from build123d import *

# Parameters (mm, degrees)
F0_W      = 78
F0_H      = 50.8
F1_DEPTH  = 38
F3_DEPTH  = 3
F5_DEPTH  = 50.8
F7_DEPTH  = 4.5
F8_R      = 1.5
F9_DEPTH  = 5
F10_W     = 3
F10_H     = 3.25
F11_DEPTH = 4.5
F12_R     = 6
F13_DEPTH = 51
F15_DEPTH = 3
F16_W     = 48.5
F16_H     = 22
F17_DEPTH = 38
F18_SIZE  = 3
F19_R     = 1
F20_DEPTH = 8
F21_R     = 1
F22_DEPTH = 8
F23_R     = 1
F24_DEPTH = 8
F25_R     = 1
F26_DEPTH = 10


with BuildPart() as f1:
    # F0 (on Front) → F1 (new body)
    with BuildSketch(Plane.XZ):
        with Locations((39, 25.4)):
            Rectangle(F0_W, F0_H)
    extrude(amount=F1_DEPTH)

    # F2 (on face) → F3 (cut)
    with BuildSketch(Plane.XY.offset(50.8)):
        with BuildLine():
            Line((70, -2), (8, -2))
            ThreePointArc((8, -2), (6.5857864376, -2.5857864376), (6, -4))
            Line((6, -4), (6, -34))
            ThreePointArc((6, -34), (6.5857864376, -35.4142135624), (8, -36))
            Line((8, -36), (70, -36))
            ThreePointArc((70, -36), (71.4142135624, -35.4142135624), (72, -34))
            Line((72, -34), (72, -4))
            ThreePointArc((72, -4), (71.4142135624, -2.5857864376), (70, -2))
        make_face()
    extrude(amount=-F3_DEPTH, mode=Mode.SUBTRACT)

    # F4 (on face) → F5 (cut, through all)
    with BuildSketch(Plane.XY.offset(50.8)):
        with BuildLine():
            ThreePointArc((62, -2), (54.9289321881, -4.9289321881), (52, -12))
            Line((52, -12), (52, -26))
            ThreePointArc((52, -26), (54.9289321881, -33.0710678119), (62, -36))
            ThreePointArc((62, -36), (68.9507563357, -33.1893662003), (71.9943065333, -26.3373972723))
            ThreePointArc((71.9943065333, -26.3373972723), (75.2, -19), (71.9943065333, -11.6626027277))
            ThreePointArc((71.9943065333, -11.6626027277), (68.9507563357, -4.8106337997), (62, -2))
        make_face()
    extrude(amount=-F5_DEPTH, mode=Mode.SUBTRACT)

    # F6 (on face) → F7 (cut)
    with BuildSketch(Plane.XY.offset(50.8)):
        with BuildLine():
            Line((47.25, -2), (38.75, -2))
            ThreePointArc((38.75, -2), (38.0428932188, -2.2928932188), (37.75, -3))
            Line((37.75, -3), (37.75, -11.5))
            ThreePointArc((37.75, -11.5), (38.0428932188, -12.2071067812), (38.75, -12.5))
            Line((38.75, -12.5), (47.25, -12.5))
            ThreePointArc((47.25, -12.5), (47.9571067812, -12.2071067812), (48.25, -11.5))
            Line((48.25, -11.5), (48.25, -3))
            ThreePointArc((48.25, -3), (47.9571067812, -2.2928932188), (47.25, -2))
        make_face()
    extrude(amount=-F7_DEPTH, mode=Mode.SUBTRACT)

    # F8 (on face) → F9 (cut)
    with BuildSketch(Plane.XY.offset(50.8)):
        with Locations((47, -11.25)):
            Circle(F8_R)
        with Locations((39, -11.25)):
            Circle(F8_R)
        with Locations((39, -3.25)):
            Circle(F8_R)
        with Locations((47, -3.25)):
            Circle(F8_R)
    extrude(amount=-F9_DEPTH, mode=Mode.SUBTRACT)

    # F10 (on face) → F11 (cut)
    with BuildSketch(Plane.XY.offset(50.8)):
        with Locations((39, -1.625)):
            Rectangle(F10_W, F10_H)
    extrude(amount=-F11_DEPTH, mode=Mode.SUBTRACT)

    # F12 (on face) → F13 (cut)
    with BuildSketch(Plane.XY.offset(50.8)):
        with Locations((20.5, -19)):
            Circle(F12_R)
    extrude(amount=-F13_DEPTH, mode=Mode.SUBTRACT)

    # F14 (on face) → F15 (cut)
    with BuildSketch(Plane(origin=(0, 0, 0), x_dir=(1, 0, 0), z_dir=(0, 0, -1))):
        with BuildLine():
            Line((70, 36), (8, 36))
            ThreePointArc((8, 36), (6.5857864376, 35.4142135624), (6, 34))
            Line((6, 34), (6, 4))
            ThreePointArc((6, 4), (6.5857864376, 2.5857864376), (8, 2))
            Line((8, 2), (70, 2))
            ThreePointArc((70, 2), (71.4142135624, 2.5857864376), (72, 4))
            Line((72, 4), (72, 34))
            ThreePointArc((72, 34), (71.4142135624, 35.4142135624), (70, 36))
        make_face()
    extrude(amount=-F15_DEPTH, mode=Mode.SUBTRACT)

    # F16 (on face) → F17 (cut, through all)
    with BuildSketch(Plane.XZ.offset(38)):
        with Locations((24.25, 28)):
            Rectangle(F16_W, F16_H)
    extrude(amount=-F17_DEPTH, mode=Mode.SUBTRACT)

    # F18
    f18_edges = [f1.edges().sort_by_distance(p)[0] for p in [
        (0, -19, 39),
        (0, -19, 17),
    ]]
    chamfer(f18_edges, length=F18_SIZE)

    # F19 (on face) → F20 (cut)
    with BuildSketch(Plane.XY.offset(50.8)):
        with Locations((3, -19)):
            Circle(F19_R)
        with Locations((75, -10)):
            Circle(F19_R)
        with Locations((75, -28)):
            Circle(F19_R)
    extrude(amount=-F20_DEPTH, mode=Mode.SUBTRACT)

    # F21 (on face) → F22 (cut)
    with BuildSketch(Plane(origin=(0, 0, 0), x_dir=(1, 0, 0), z_dir=(0, 0, -1))):
        with Locations((75, 28)):
            Circle(F21_R)
        with Locations((75, 10)):
            Circle(F21_R)
        with Locations((3, 19)):
            Circle(F21_R)
    extrude(amount=-F22_DEPTH, mode=Mode.SUBTRACT)

    # F23 (on face) → F24 (cut)
    with BuildSketch(Plane(origin=(0, 0, 3), x_dir=(1, 0, 0), z_dir=(0, 0, -1))):
        with Locations((41.5, 15)):
            Circle(F23_R)
    extrude(amount=-F24_DEPTH, mode=Mode.SUBTRACT)

    # F25 (on face) → F26 (cut)
    with BuildSketch(Plane.YZ.offset(78)):
        with Locations((-26.7781745931, 34.7781745931)):
            Circle(F25_R)
        with Locations((-11.2218254069, 34.7781745931)):
            Circle(F25_R)
        with Locations((-26.7781745931, 19.2218254069)):
            Circle(F25_R)
        with Locations((-11.2218254069, 19.2218254069)):
            Circle(F25_R)
    extrude(amount=-F26_DEPTH, mode=Mode.SUBTRACT)


solid = f1.part
Geometry: final body of the model. Coordinates: model frame, mm. A direction names the side the tool comes from. Coordinates: 2 decimals unless noted, no trailing zeros. Loops run counter-clockwise (first coordinate to the right, second up) from the corner with the lowest first, then second, coordinate; pieces in that order, holes last. Notation, with made-up numbers: M 25,-25.5 L 32,-25.5 A20 cw 32,-3.5 Z; hole C 58.25,-40 d1. An arc over 180 degrees is marked long. One line per item, written item: value. Start each with the question number.
1) Draft query along Y for faces 5 (the flat face through (6, -19, 1)), 6 (the flat face through (0, -19, 7)). Return one class per face: released by +Y, released by -Y, zero draft, split by the parting line, or undercut.
2) Cut plane C-C (y = -30). Return loops of the section in (x, z), then the cut area to 3 significant figures.
3) Material intervals for L1, parallel to Y at x = 39, z = 46; L2, parallel to Z at x = 47.5, y = -10; L3, parallel to X at y = -28, z = 4, sorted ascending. Write a range as from..to.
4) Pin query (flat end, axial travel): P1, Ø6, axis at y = -22.5, z = 18.5, coming from the -X side; P2, Ø1, axis at x = 28, z = 45.5, coming from the +Y side; P3, Ø1.5, axis at x = 39, y = -11, coming from the +Z side; P4, Ø3, axis at x = 45, y = -5, coming from the +Z side. Return the tip coordinate at first contact, or that it passes through.
5) Reachability of faces 1 (the flat face through (70, -4, 47.8)), 2 (the flat face through (25.4, -23.5, 17)), 3 (the flat face through (40.5, -1, 49)), 4 (the flat face through (72, -30, 1)) from +Z, -Z, +X, -X, +Y, -Y: full face, straight path, thin tool, end or side. Return the list, or none.
6) Cut plane A-A (x = 47). Return loops of the section in (y, z).
7) Cut plane D-D (x = 20.5). Return loops of the section in (y, z), then the cut area to 3 significant figures.
Evaluation:
1. face 5: undercut
1. face 6: zero draft
2. outline: M 0,0 L 6,0 L 6,3 L 52.83,3 L 52.83,47.8 L 6,47.8 L 6,50.8 L 0,50.8 L 0,42 L 3,39 L 48.5,39 L 48.5,17 L 3,17 L 0,14 Z; M 71.17,3 L 72,3 L 72,0 L 78,0 L 78,50.8 L 72,50.8 L 72,47.8 L 71.17,47.8 Z
2. area: 1,670 mm^2
3. L1: -38..-12.75, -9.75..-4.75, -1.75..0
3. L2: 3..17, 39..45.8
3. L3: 0..52.2, 71.8..74, 76..78
4. P1: x = 1.5
4. P2: y = 0
4. P3: z = 45.8
4. P4: z = 46.3
5. face 1: +Z
5. face 2: -X, +Y, -Y
5. face 3: +Z, +Y
5. face 4: -Z
6. outline: M -38,0 L -36,0 L -36,3 L -2,3 L -2,0 L 0,0 L 0,17 L -38,17 Z; M -38,39 L 0,39 L 0,50.8 L -1.75,50.8 L -1.75,45.8 L -4.75,45.8 L -4.75,46.3 L -9.75,46.3 L -9.75,45.8 L -12.75,45.8 L -12.75,47.8 L -36,47.8 L -36,50.8 L -38,50.8 Z
7. outline: M -38,0 L -36,0 L -36,3 L -25,3 L -25,17 L -38,17 Z; M -38,39 L -25,39 L -25,47.8 L -36,47.8 L -36,50.8 L -38,50.8 Z; M -13,3 L -2,3 L -2,0 L 0,0 L 0,17 L -13,17 Z; M -13,39 L 0,39 L 0,50.8 L -2,50.8 L -2,47.8 L -13,47.8 Z
7. area: 617 mm^2
